The figure shows three views and two pictorial views of one solid part (mm, origin at its lowest corner). Answer the questions. Give positions to 0.01 mm unless a question says otherwise; leave off trailing zeros. Write each loop counter-clockwise with the first axis right and the second up, starting at its lowest first coordinate (ties: lowest second). Pieces come first, ordered by that corner, then holes. Notation, with made-up numbers: (89, 60) - (132, 60) arc R24 cw to (132, 80) - close; hole circle Ø2 at (88, 34). An arc over 180 degrees is marked (long way). One line per question, with ' | ' between items. Start each with the question number.
1. A cutting plane is placed at C-C (y = 4). Determine the outline of the cut face in (x, z).
2. A cutting plane is placed at B-B (x = 50). Determine the outline of the cut face in (y, z).
3. The mould has two halves that part along X. Classify the marked faces 1, 2 and 3: +X half, -X half, draft (parallel to the pull), parting line (faces both ways), or undercut.
4. A cutting plane is placed at D-D (x = 6). Determine the outline of the cut face in (y, z).
5. A cutting plane is placed at A-A (x = 72). Determine the outline of the cut face in (y, z).
6. Find the intervals of material crossed by L1, parallel to Z at x = 72, y = 6.25; L2, parallel to Y at x = 35, z = 44; L3, parallel to X at y = 11.25, z = 49 (1 decimal), in increasing order. Write a range as from..to.
7. Given P1, Ø5, axis at y = 4.5, z = 14, coming from the +X side; P2, Ø3, axis at y = 3.5, z = 51, coming from the +X side; P3, Ø1.5, axis at y = 9, z = 77, coming from the -X side, each flat-ended and moving along its own axis, determine where each tip first touches the part or whether it passes through.
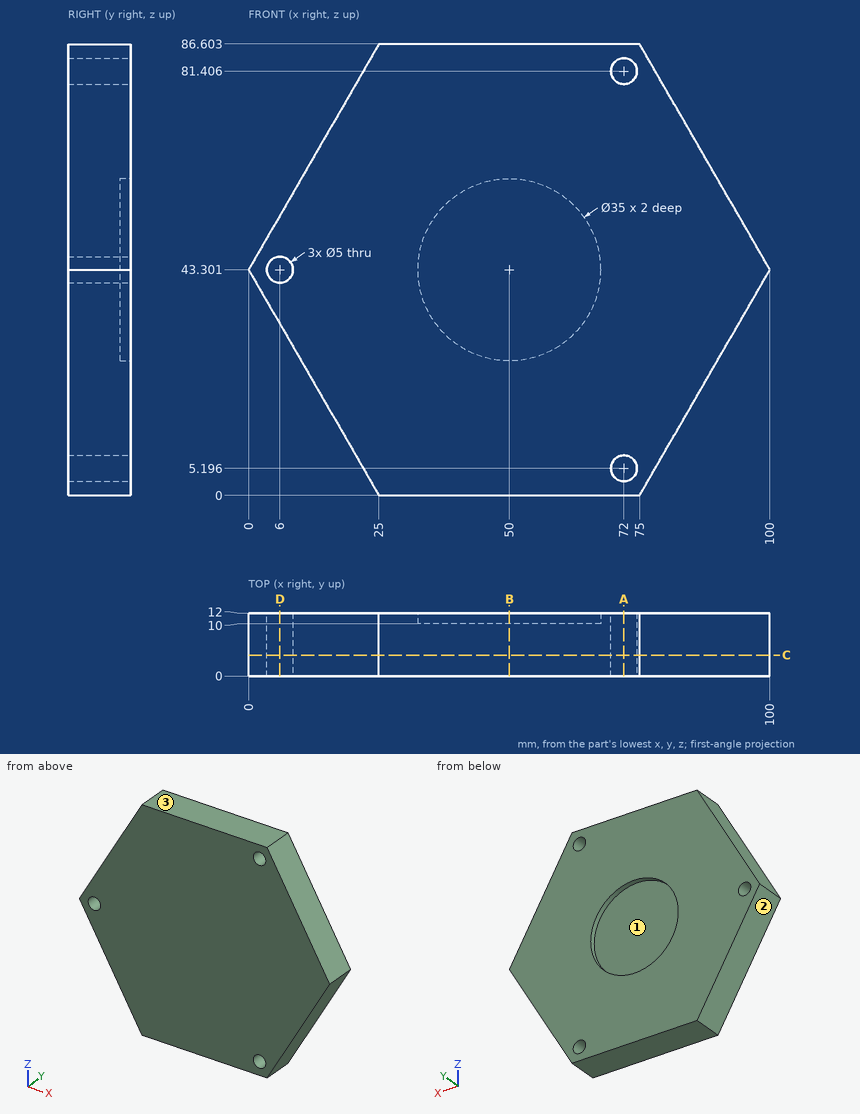
Determined:
1) outline: (0, 43.3) - (25, 0) - (75, 0) - (100, 43.3) - (75, 86.6) - (25, 86.6) - close; hole circle Ø5 at (6, 43.3); hole circle Ø5 at (72, 5.2); hole circle Ø5 at (72, 81.41)
2) outline: (0, 0) - (12, 0) - (12, 25.8) - (10, 25.8) - (10, 60.8) - (12, 60.8) - (12, 86.6) - (0, 86.6) - close
3) face 1: undercut | face 2: -X half | face 3: draft
4) outline: (0, 32.91) - (12, 32.91) - (12, 40.8) - (0, 40.8) - close; (0, 45.8) - (12, 45.8) - (12, 53.69) - (0, 53.69) - close
5) outline: (0, 0) - (12, 0) - (12, 2.7) - (0, 2.7) - close; (0, 7.7) - (12, 7.7) - (12, 78.91) - (0, 78.91) - close; (0, 83.91) - (12, 83.91) - (12, 86.6) - (0, 86.6) - close
6) L1: 0..2.7, 7.7..78.91, 83.91..86.6 | L2: 0..10 | L3: 3.3..33.5, 66.5..96.7
7) P1: x = 84.53 | P2: x = 96.42 | P3: x = 19.02
